Geometry check sheet. Reference: the model listing, model coordinates, mm. A direction names the side the tool comes from. Give positions to 0.01 mm unless a question says otherwise; leave off trailing zeros. Order: outer loops, then holes, each group sorted by start corner. A loop starts at its lowest first (then second) coordinate and runs counter-clockwise, first axis right, second up. Notation, with made-up numbers: M 13.5,32 L 33.5,32 A26 cw 33.5,53 Z; hole C 30,17 d10. An arc over 180 degrees is marked long. Put each result on its own line as item: value. Start each with the question number.
Q1. Go/stop test with flat-tipped pins: pin 1 (1.7 mm diameter, centred on x = -6.58, y = 2.39, fed in from -Z); pin 2 (3 mm diameter, centred on x = 8, z = 2, fed in from +Y); pin 3 (4 mm diameter, centred on x = -2.5, y = -8.5, fed in from +Z). Record where each tip stops, or that it passes through.
Q2. Access from +Z, -Z, +X, -X, +Y, -Y to the whole of each face (thin tool, end or side, straight path). Record for faces 1 (the cylindrical face through (-11.99, -0.53, 0.99)), 2 (the cylindrical face through (-0.59, 4.46, -1.23)), 3 (the flat face through (-3, 3, 2)).
Q3. Section check D-D on x = -7. Record the cut outline in (y, z).
Q4. Section check B-B on z = -0.45. Record the cut outline in (x, y), then the cut area to 3 significant figures.
Q5. Material ranges on L1, parallel to X at y = 0, z = 1.5; L2, parallel to X at y = 0, z = 1; L3, parallel to Y at x = 0, z = 1.1, recorded low to high.
Q6. Section check C-C on y = -8.25. Record the cut outline in (x, z), then the cut area to 3 significant figures.
Q7. Mould release check, pull along Y, two halves, no side actions. Record for faces 4 (the cylindrical face through (7.732, -0.163, 1.014)), 5 (the cylindrical face through (-3.414, -8.54, 1.014)), 6 (the flat face through (1, -3, -2.5)), 7 (the cylindrical face through (-3.746, -0.165, 2.246)): +Y half, -Y half, draft (parallel to the pull), parting line (faces both ways), or undercut.
Q8. Section check A-A on x = 0. State how many separate pieces and enclosed holes the cut face has, then the cut area to 3 significant figures.
Autodesk Inventor part; units mm, degrees
ref_plane "YZ Plane" through (0, 0, 0) normal (1, 0, 0) x (0, 1, 0)
ref_plane "XZ Plane" through (0, 0, 0) normal (0, 1, 0) x (-1, 0, 0)
ref_plane "XY Plane" through (0, 0, 0) normal (0, 0, 1) x (1, 0, 0)
sketch "Sketch1" plane through (0, 0, 0) normal (0, 0, 1) x (1, 0, 0)
  line L0 (-16.8, 0) -> (16.8, 0)
  line L1 (0, 16.8) -> (0, -16.8)
  circle A0 centre (0, 0) radius 12
  dimension "d0" = 24
extrude "Extrusion1" add sketch "Sketch1" along normal blind 2
sketch "Sketch2" plane through (0, 0, 0) normal (0, 0, 1) x (1, 0, 0)
  line L0 (0, 16.8) -> (0, -16.8)
  line L1 (-16.8, 0) -> (16.8, 0)
  circle A0 centre (0, 0) radius 4.5
  dimension "d3" = 9
extrude "Extrusion2" add sketch "Sketch2" against normal blind 2.5
sketch "Sketch3" plane through (0, 0, -2.5) normal (0, 0, -1) x (-1, 0, 0)
  line L0 (-16.8, 0) -> (16.8, 0)
  line L1 (0, -16.8) -> (0, 16.8)
  circle A0 centre (0, 0) radius 2.9
  dimension "d6" = 5.8
extrude "Extrusion3" cut sketch "Sketch3" against normal blind 3
sketch "Sketch4" plane through (0, 0, 2) normal (0, 0, 1) x (1, 0, 0)
  line L0 (0, 16.8) -> (0, -16.8)
  line L1 (-16.8, 0) -> (16.8, 0)
  circle A0 centre (0, 0) radius 3.75
  dimension "d9" = 7.5
extrude "Extrusion4" add sketch "Sketch4" along normal blind 0.5
sketch "Sketch5" plane through (0, 0, 2.5) normal (0, 0, 1) x (1, 0, 0)
  line L0 (0, 16.8) -> (0, -16.8)
  line L1 (-16.8, 0) -> (16.8, 0)
  circle A0 centre (0, 0) radius 3
  dimension "d12" = 6
extrude "Extrusion5" cut sketch "Sketch5" against normal blind 1.2
sketch "Sketch6" plane through (0, 0, 0) normal (0, 0, 1) x (1, 0, 0)
  line L0 (0, 16.8) -> (0, -16.8)
  line L1 (-16.8, 0) -> (16.8, 0)
  circle A0 centre (0, 0) radius 1.4
  dimension "d15" = 2.8
extrude "Extrusion6" cut sketch "Sketch6" along normal through all
sketch "Sketch7" plane through (0, 0, 0) normal (0, 0, 1) x (1, 0, 0)
  line L0 (0, 16.8) -> (0, -16.8)
  line L1 (-16.8, 0) -> (16.8, 0)
  circle A0 centre (0, 0) radius 8.5 construction
  line L2 (-2.9072, 7.9874) -> (2.9072, -7.9874) construction
  line L3 (2.9072, 7.9874) -> (-2.9072, -7.9874) construction
  point P0 (0, 8.5)
  point P1 (0, -8.5)
  dimension "d18" = 17
  dimension "d20" = 20
hole "Hole1" at (0, 8.5, 0) at (0, -8.5, 0) at (2.9072, 7.9874, 0) at (-2.9072, 7.9874, 0) at (2.9072, -7.9874, 0) at (-2.9072, -7.9874, 0) direction (0, 0, 1) diameter 1.5 depth 8 tip angle 118
sketch "Sketch8" plane through (0, 0, 0) normal (0, 0, 1) x (1, 0, 0)
  line L0 (0, 16.8) -> (0, -16.8)
  line L1 (-16.8, 0) -> (16.8, 0)
  circle A0 centre (0, 0) radius 10 construction
  line L2 (9.3969, 3.4202) -> (-9.3969, -3.4202) construction
  line L3 (-9.3969, 3.4202) -> (9.3969, -3.4202) construction
  circle A1 centre (0, 0) radius 7 construction
  point P0 (-10, 0)
  point P1 (10, 0)
  point P2 (-6.5778, 2.3941)
  point P3 (-7, 0)
  point P4 (-6.5778, -2.3941)
  point P5 (6.5778, 2.3941)
  point P6 (7, 0)
  point P7 (6.5778, -2.3941)
  dimension "d28" = 20
  dimension "d30" = 40
  dimension "d31" = 14
hole "Hole2" at (-10, 0, 0) at (-9.3969, 3.4202, 0) at (-9.3969, -3.4202, 0) at (10, 0, 0) at (9.3969, 3.4202, 0) at (9.3969, -3.4202, 0) at (-6.5778, 2.3941, 0) at (-7, 0, 0) at (-6.5778, -2.3941, 0) at (6.5778, 2.3941, 0) at (7, 0, 0) at (6.5778, -2.3941, 0) direction (0, 0, 1) diameter 1.5 depth 8 tip angle 118
properties part number "servo motor HS-7955TG round horn"
Results found:
1. pin 1: stops at z = 0
1. pin 2: stops at y = 10.09
1. pin 3: stops at z = 2
2. face 1: +Z, -Z
2. face 2: -Z
2. face 3: +Z
3. outline: M -9.75,0 L -3.01,0 L -3.01,2 L -9.75,2 Z; M -1.77,0 L -0.75,0 L -0.75,2 L -1.77,2 Z; M 0.75,0 L 1.77,0 L 1.77,2 L 0.75,2 Z; M 3.01,0 L 9.75,0 L 9.75,2 L 3.01,2 Z
4. outline: C 0,0 d9; hole C 0,0 d5.8
4. area: 37.2 mm^2
5. L1: x = -12 to -10.75, -9.25 to -7.75, -6.25 to -3, 3 to 6.25, 7.75 to 9.25, 10.75 to 12
5. L2: x = -12 to -10.75, -9.25 to -7.75, -6.25 to -1.4, 1.4 to 6.25, 7.75 to 9.25, 10.75 to 12
5. L3: y = -12 to -9.25, -7.75 to -1.4, 1.4 to 7.75, 9.25 to 12
6. outline: M -8.71,0 L -3.61,0 L -3.61,2 L -8.71,2 Z; M -2.2,0 L -0.71,0 L -0.71,2 L -2.2,2 Z; M 0.71,0 L 2.2,0 L 2.2,2 L 0.71,2 Z; M 3.61,0 L 8.71,0 L 8.71,2 L 3.61,2 Z
6. area: 26.4 mm^2
7. face 4: undercut
7. face 5: undercut
7. face 6: draft
7. face 7: parting line
8. separate pieces: 4
8. enclosed holes: 0
8. area: 41.4 mm^2
